Here's how the part is built. I have some questions about the finished solid (model axes, mm). Face numbers are marked on the shaded views. A direction names the side the tool comes from. Coordinates: 2 decimals unless noted, no trailing zeros. Write each loop counter-clockwise with the first axis right and the second up, starting at its lowest first coordinate (ties: lowest second). Pieces come first, ordered by that corner, then holes.
Item 1: I'm going to push flat-ended pins straight in: pin 1 Ø0.9 at (y, z) = (1, -41.5) entering from -X; pin 2 Ø5 at (y, z) = (20.5, -64) entering from +X; pin 3 Ø10 at (x, z) = (20.5, -40) entering from -Y. Where does each tip first touch, or does it pass through?
Item 2: For the marked faces 4 and 5, which set-ups out of +Z, -Z, +X, -X, +Y, -Y let a thin tool reach every point of the face, with its end or its side?
Item 3: If I drill on line 1 (X direction, y = 34, z = -70); line 2 (X direction, y = 4, z = -4); line 3 (Y direction, x = 7, z = -14), over which ranges is the centre line in solid material (lowest first)?
Item 4: If we section it at D-D (x = 74): Please give me the cut outline in (y, z).
Item 5: If we section it at C-C (y = 22): Please give me the cut outline in (x, z), then the cut area to 3 significant figures.
Item 6: We'd pull the mould along Z, two halves only. Please class the marked faces 1, 2 and 3: +Z half, -Z half, draft (parallel to the pull), parting line (faces both ways), or undercut.
Item 7: If we section it at A-A (z = -38): Please give me the cut outline in (x, y).
Item 8: If we section it at B-B (x = 30.5): Please give me the cut outline in (y, z), then the cut area to 3 significant figures.
from build123d import *

# Parameters (mm, degrees)
SKETCH1_W                             = 66
SKETCH1_H                             = 74
SKETCH1_R                             = 1.2
MAIN_OUTER_CONNECTION_DEPTH           = 40
SKETCH2_W                             = 62
SKETCH2_H                             = 30
HOLE_FOR_PROTOBOARD_ACCESS_DEPTH      = 107.920531237
SKETCH16_W                            = 5
SKETCH16_H                            = 30
WALL_FOR_SCREW_TERMINAL_REPLACE_DEPTH = 2
SKETCH18_W                            = 58
SKETCH18_H                            = 30
HOLE_FOR_WIRE_CONNECTIONS_DEPTH       = 107.920531237
HOLE_FOR_SCREW_TERMINAL_REPLACE_REACH = 108.921
SKETCH18_3_W                          = 5
SKETCH18_3_H                          = 30
SKETCH1_3_W                           = 6
SKETCH1_3_H                           = 46
HOLE_FOR_WIRE_IN_BOTTOM_DEPTH         = 10
BOLT_START                            = 33
SKETCH1_5_R                           = 3.2
SKETCH1_5_R_2                         = 1.2
BOLT_HEAD_CLEARANCE_DEPTH             = 7
STANDOFF_START                        = 3
SKETCH1_6_R                           = 3.2
SKETCH1_6_R_2                         = 1.2
STANDOFF_FOR_WIRE_CLEARANCE_DEPTH     = 3
BREAKOUT_START                        = 36
SKETCH1_8_W                           = 15
SKETCH1_8_H                           = 30
BREAKOUT_BOARD_COVER_DEPTH            = 4
CUT_EXTRUDE14_START                   = 40
SKETCH1_9_W                           = 5
SKETCH1_9_H                           = 15
CUT_EXTRUDE14_DEPTH                   = 7
CHAMFER2_SIZE                         = 6


with BuildPart() as part:
    # Sketch1 → Main Outer Connection (new body)
    with BuildSketch(Plane(origin=(0, 0, 0), x_dir=(1, 0, 0), z_dir=(0, 1, 0))):
        with Locations((33, 37)):
            Rectangle(SKETCH1_W, SKETCH1_H)
        with Locations(Location((10, 70, 0), (0, 0, 270))):
            Circle(SKETCH1_R, mode=Mode.SUBTRACT)
        with Locations(Location((56, 70, 0), (0, 0, 270))):
            Circle(SKETCH1_R, mode=Mode.SUBTRACT)
        with Locations(Location((10, 4, 0), (0, 0, 270))):
            Circle(SKETCH1_R, mode=Mode.SUBTRACT)
        with Locations(Location((56, 4, 0), (0, 0, 270))):
            Circle(SKETCH1_R, mode=Mode.SUBTRACT)
    extrude(amount=MAIN_OUTER_CONNECTION_DEPTH)

    # Sketch2 → Hole for Protoboard Access (cut, through all)
    with BuildSketch(Plane(origin=(0, 0, -74), x_dir=(-1, 0, 0), z_dir=(0, 0, -1))):
        with Locations((-33, 18)):
            Rectangle(SKETCH2_W, SKETCH2_H)
    extrude(amount=-HOLE_FOR_PROTOBOARD_ACCESS_DEPTH, mode=Mode.SUBTRACT)

    # Sketch16 → Wall for Screw Terminal Replace (add)
    with BuildSketch(Plane.XY):
        with Locations((61.5, 18)):
            Rectangle(SKETCH16_W, SKETCH16_H)
        with Locations((4.5, 18)):
            Rectangle(SKETCH16_W, SKETCH16_H)
    extrude(amount=-WALL_FOR_SCREW_TERMINAL_REPLACE_DEPTH)

    # Sketch18 → Hole for Wire Connections (cut, through all)
    with BuildSketch(Plane(origin=(66, 0, 0), x_dir=(0, 0, -1), z_dir=(1, 0, 0))):
        with Locations((37, 18)):
            Rectangle(SKETCH18_W, SKETCH18_H)
    extrude(amount=-HOLE_FOR_WIRE_CONNECTIONS_DEPTH, mode=Mode.SUBTRACT)

    # Sketch18<3> → Hole for Screw Terminal Replace (cut, up to next)
    with BuildSketch(Plane(origin=(66, 0, 0), x_dir=(0, 0, -1), z_dir=(1, 0, 0)), mode=Mode.PRIVATE) as hole_for_screw_terminal_replace_sk1:
        with Locations((5.5, 18)):
            Rectangle(SKETCH18_3_W, SKETCH18_3_H)
    hole_for_screw_terminal_replace_tool1 = extrude(hole_for_screw_terminal_replace_sk1.sketch, amount=-HOLE_FOR_SCREW_TERMINAL_REPLACE_REACH, mode=Mode.PRIVATE) & part.part
    add(hole_for_screw_terminal_replace_tool1.solids().sort_by_distance((66, 18, -5.5))[0], mode=Mode.SUBTRACT)

    # Sketch1<3> → Hole for Wire in Bottom (cut)
    with BuildSketch(Plane(origin=(0, 0, 0), x_dir=(1, 0, 0), z_dir=(0, 1, 0))):
        with Locations((3, 37)):
            Rectangle(SKETCH1_3_W, SKETCH1_3_H)
        with BuildLine():
            Line((51, 70), (15, 70))
            ThreePointArc((15, 70), (13.535533906, 66.464466094), (10, 65))
            Line((10, 65), (10, 9))
            ThreePointArc((10, 9), (13.535533906, 7.535533906), (15, 4))
            Line((15, 4), (51, 4))
            ThreePointArc((51, 4), (52.464466094, 7.535533906), (56, 9))
            Line((56, 9), (56, 65))
            ThreePointArc((56, 65), (52.464466094, 66.464466094), (51, 70))
        make_face()
    extrude(amount=HOLE_FOR_WIRE_IN_BOTTOM_DEPTH, mode=Mode.SUBTRACT)

    # Sketch1<5> → Bolt Head Clearance (cut)
    # profile 1 of 4: a face of its own
    with BuildSketch(Plane(origin=(0, 0, 0), x_dir=(1, 0, 0), z_dir=(0, 1, 0)).offset(BOLT_START)):
        with Locations(Location((56, 4, 0), (0, 0, 270))):
            Circle(SKETCH1_5_R)
        with Locations(Location((56, 4, 0), (0, 0, 90))):
            Circle(SKETCH1_5_R_2, mode=Mode.SUBTRACT)
    # profile 2 of 4: a face of its own
    with BuildSketch(Plane(origin=(0, 0, 0), x_dir=(1, 0, 0), z_dir=(0, 1, 0)).offset(BOLT_START)):
        with Locations(Location((10, 4, 0), (0, 0, 270))):
            Circle(SKETCH1_5_R)
        with Locations(Location((10, 4, 0), (0, 0, 90))):
            Circle(SKETCH1_5_R_2, mode=Mode.SUBTRACT)
    # profile 3 of 4: a face of its own
    with BuildSketch(Plane(origin=(0, 0, 0), x_dir=(1, 0, 0), z_dir=(0, 1, 0)).offset(BOLT_START)):
        with Locations(Location((10, 70, 0), (0, 0, 270))):
            Circle(SKETCH1_5_R)
        with Locations(Location((10, 70, 0), (0, 0, 90))):
            Circle(SKETCH1_5_R_2, mode=Mode.SUBTRACT)
    # profile 4 of 4: a face of its own
    with BuildSketch(Plane(origin=(0, 0, 0), x_dir=(1, 0, 0), z_dir=(0, 1, 0)).offset(BOLT_START)):
        with Locations(Location((56, 70, 0), (0, 0, 270))):
            Circle(SKETCH1_5_R)
        with Locations(Location((56, 70, 0), (0, 0, 90))):
            Circle(SKETCH1_5_R_2, mode=Mode.SUBTRACT)
    extrude(amount=BOLT_HEAD_CLEARANCE_DEPTH, mode=Mode.SUBTRACT)

    # Sketch1<6> → Standoff for Wire Clearance (add)
    # profile 1 of 4: a face of its own
    with BuildSketch(Plane(origin=(0, 0, 0), x_dir=(1, 0, 0), z_dir=(0, 1, 0)).offset(STANDOFF_START)):
        with Locations(Location((10, 4, 0), (0, 0, 270))):
            Circle(SKETCH1_6_R)
        with Locations(Location((10, 4, 0), (0, 0, 90))):
            Circle(SKETCH1_6_R_2, mode=Mode.SUBTRACT)
    # profile 2 of 4: a face of its own
    with BuildSketch(Plane(origin=(0, 0, 0), x_dir=(1, 0, 0), z_dir=(0, 1, 0)).offset(STANDOFF_START)):
        with Locations(Location((56, 4, 0), (0, 0, 270))):
            Circle(SKETCH1_6_R)
        with Locations(Location((56, 4, 0), (0, 0, 90))):
            Circle(SKETCH1_6_R_2, mode=Mode.SUBTRACT)
    # profile 3 of 4: a face of its own
    with BuildSketch(Plane(origin=(0, 0, 0), x_dir=(1, 0, 0), z_dir=(0, 1, 0)).offset(STANDOFF_START)):
        with Locations(Location((56, 70, 0), (0, 0, 270))):
            Circle(SKETCH1_6_R)
        with Locations(Location((56, 70, 0), (0, 0, 90))):
            Circle(SKETCH1_6_R_2, mode=Mode.SUBTRACT)
    # profile 4 of 4: a face of its own
    with BuildSketch(Plane(origin=(0, 0, 0), x_dir=(1, 0, 0), z_dir=(0, 1, 0)).offset(STANDOFF_START)):
        with Locations(Location((10, 70, 0), (0, 0, 270))):
            Circle(SKETCH1_6_R)
        with Locations(Location((10, 70, 0), (0, 0, 90))):
            Circle(SKETCH1_6_R_2, mode=Mode.SUBTRACT)
    extrude(amount=STANDOFF_FOR_WIRE_CLEARANCE_DEPTH)

    # Sketch1<8> → Breakout Board Cover (add)
    with BuildSketch(Plane(origin=(0, 0, 0), x_dir=(1, 0, 0), z_dir=(0, 1, 0)).offset(BREAKOUT_START)):
        with Locations((73.5, 39)):
            Rectangle(SKETCH1_8_W, SKETCH1_8_H)
    extrude(amount=BREAKOUT_BOARD_COVER_DEPTH)

    # Sketch1<9> → Cut-Extrude14 (cut)
    with BuildSketch(Plane(origin=(0, 0, 0), x_dir=(1, 0, 0), z_dir=(0, 1, 0)).offset(CUT_EXTRUDE14_START)):
        with Locations((51.5, 56.5)):
            Rectangle(SKETCH1_9_W, SKETCH1_9_H)
    extrude(amount=-CUT_EXTRUDE14_DEPTH, mode=Mode.SUBTRACT)

    # Chamfer2
    chamfer2_edges = [part.edges().sort_by_distance(p)[0] for p in [
        (66, 38, -24),
        (66, 38, -54),
    ]]
    chamfer(chamfer2_edges, length=CHAMFER2_SIZE)


solid = part.part
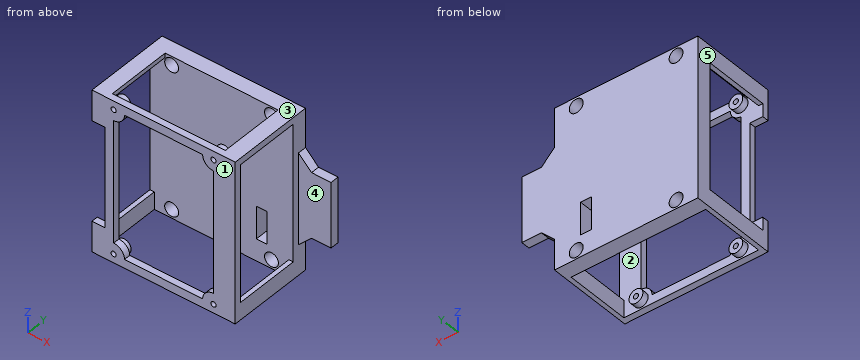
Answer list:
1. pin 1: stops at x = 6
1. pin 2: stops at x = 66
1. pin 3: stops at y = 33
2. face 4: +Z, -Z, +X, -Y
2. face 5: +Z, -Z, -X, +Y, -Y
3. line 1: x = 0 to 6.8, 13.2 to 52.8, 59.2 to 66
3. line 2: x = 0 to 2, 6.8 to 8.8, 11.2 to 13.2, 52.8 to 54.8, 57.2 to 59.2
3. line 3: y = 0 to 3, 33 to 40
4. outline: (36, -54) - (40, -54) - (40, -24) - (36, -24) - close
5. outline: (0, -74) - (2, -74) - (2, -66) - (0, -66) - close; (0, -8) - (2, -8) - (2, -2) - (7, -2) - (7, 0) - (0, 0) - close; (59, -2) - (64, -2) - (64, -3) - (66, -3) - (66, 0) - (59, 0) - close; (64, -74) - (66, -74) - (66, -66) - (64, -66) - close
5. area: 74.0 mm2
6. face 1: draft
6. face 2: undercut
6. face 3: +Z half
7. outline: (0, 33) - (66, 33) - (66, 36) - (81, 36) - (81, 40) - (0, 40) - close; (6, 0) - (10, 0) - (10, 3) - (6, 3) - close; (56, 0) - (66, 0) - (66, 3) - (56, 3) - close
8. outline: (0, -74) - (3, -74) - (3, -70) - (0, -70) - close; (0, -4) - (3, -4) - (3, 0) - (0, 0) - close; (33, -74) - (40, -74) - (40, 0) - (33, 0) - close
8. area: 542 mm2
